Verification items for the finished model (mm, model axes). Give positions to 0.01 mm unless a question says otherwise; leave off trailing zeros. Loops run counter-clockwise (first coordinate to the right, second up) from the corner with the lowest first, then second, coordinate; pieces in that order, holes last. Notation, with made-up numbers: (43.5, 58) - (93.5, 58) arc R19 cw to (93.5, 95) - close; hole circle Ø6 at (-3, 67.5). An arc over 180 degrees is marked (long way). One line per question, with ' | ' between items. Start each with the question number.
1. Depth check by flat-ended pin: pin 1 Ø1.5 at (x, z) = (-42.5, -1) entering from +Y; pin 2 Ø9 at (x, y) = (-34, -12.5) entering from -Z; pin 3 Ø3 at (x, z) = (49.5, -3) entering from -Y. Enter the tip coordinate at first touch or a pass-through.
2. Section check D-D, the plane y = -13.5. Enter the section's corners in (x, z).
3. Section check B-B, the plane x = -34. Enter the section's corners in (y, z).
4. Section check A-A, the plane y = -22.5. Enter the section's corners in (x, z), then the cut area to 3 significant figures.
5. Section check C-C, the plane z = -2. Enter the section's corners in (x, y), then the cut area to 3 significant figures.
6. Thickness scan on line 1 along Y through (x, z) = (59.5, 0.85); line 2 along X through (y, z) = (-12.5, 1.55); line 3 along X through (y, z) = (-34.5, 1.4). Record the ranges inside material, lowest first. Write a range as from..to.
7. Mould release check, pull along Y, two halves, no side actions. Record for faces 1 (the face through (-60.933, 33.586, 0.986)), 2 (the face through (-1, -8, 0)), 3 (the face through (-36.77, -12.14, 0.99)), 4 (the face through (53.692, -7.663, -2.465)): +Y half, -Y half, draft (parallel to the pull), parting line (faces both ways), or undercut.
Autodesk Inventor part; units mm, degrees
ref_plane "YZ Plane" through (0, 0, 0) normal (1, 0, 0) x (0, 1, 0)
ref_plane "XZ Plane" through (0, 0, 0) normal (0, 1, 0) x (-1, 0, 0)
ref_plane "XY Plane" through (0, 0, 0) normal (0, 0, 1) x (1, 0, 0)
sketch "Sketch1" plane through (0, 0, 0) normal (0, 0, 1) x (1, 0, 0)
  line L0 (-62.5, 37.5) -> (62.5, 37.5)
  line L1 (62.5, 37.5) -> (62.5, -37.5)
  line L2 (62.5, -37.5) -> (-62.5, -37.5)
  line L3 (-62.5, -37.5) -> (-62.5, 37.5)
  point P0 (0, 0)
  point P1 (-62.5, 0)
  point P2 (0, 37.5)
  dimension "d0" = 125
  dimension "d1" = 75
extrude "Extrusion1" add sketch "Sketch1" along normal blind 2
sketch "Sketch2" plane through (0, 0, 2) normal (0, 0, 1) x (1, 0, 0)
  line L0 (-62.5, -37.5) -> (62.5, -37.5)
  line L1 (62.5, -37.5) -> (62.5, 37.5)
  line L2 (62.5, 37.5) -> (-62.5, 37.5)
  line L3 (-62.5, 37.5) -> (-62.5, -37.5)
  line L4 (-59.5, 34.5) -> (59.5, 34.5)
  line L5 (59.5, 34.5) -> (59.5, -34.5)
  line L6 (59.5, -34.5) -> (-59.5, -34.5)
  line L7 (-59.5, -34.5) -> (-59.5, 34.5)
  point P0 (0, 0)
  dimension "d4" = 3
hole "Hole1" at (-59.5, 34.5, 2) at (59.5, 34.5, 2) at (-59.5, -34.5, 2) at (59.5, -34.5, 2) direction (0, 0, -1) diameter 3.4 end through all
fillet "Fillet1" radius 2 4 edges at (-62.5, 37.5, 1) (-62.5, -37.5, 1) (62.5, -37.5, 1) (62.5, 37.5, 1)
sketch "Sketch3" plane through (0, 0, 2) normal (0, 0, 1) x (1, 0, 0)
  line L0 (18.5, 12.5) -> (45.5, 12.5)
  line L1 (45.5, 12.5) -> (45.5, -27.5)
  line L2 (45.5, -27.5) -> (18.5, -27.5)
  line L3 (18.5, -27.5) -> (18.5, 12.5)
  line L4 (62.5, -35.5) -> (62.5, 35.5)
  line L5 (60.5, 37.5) -> (-60.5, 37.5)
  point P0 (0, 0)
  dimension "d13" = 27
  dimension "d14" = 40
  dimension "d16" = 17
  dimension "d73" = 25
extrude "Extrusion2" cut sketch "Sketch3" against normal through all
fillet "Fillet2" radius 1.5 4 edges at (18.5, -27.5, 1) (18.5, 12.5, 1) (45.5, 12.5, 1) (45.5, -27.5, 1)
sketch "Sketch4" plane through (0, 0, 2) normal (0, 0, 1) x (1, 0, 0)
  line L0 (44, 12.5) -> (20, 12.5)
  line L1 (44, -27.5) -> (20, -27.5)
  line L2 (18.5, -26) -> (18.5, 11)
  line L3 (20, 12.5) -> (44, 12.5)
  line L4 (45.5, 11) -> (45.5, -26)
  line L5 (14.0041, -17.1435) -> (14.0041, 2.1435)
  line L6 (49.9959, 2.1435) -> (49.9959, -17.1435)
  line L7 (32, 12.5) -> (32, -27.5)
  point P0 (0, 0)
  point P1 (14.0041, -7.5)
  point P2 (49.9959, -7.5)
  point P3 (18.5, -7.5)
  point P4 (45.5, -7.5)
  dimension "d21" = 35.9918
hole "Hole2" at (14.0041, -7.5, 2) at (49.9959, -7.5, 2) direction (0, 0, -1) diameter 3.4 depth 6 tip angle 118
sketch "Sketch6" plane through (0, 0, 2) normal (0, 0, 1) x (1, 0, 0)
  circle A0 centre (-0.5, 10.5) radius 12.75
  line L0 (-11.4, 17.1146) -> (-11.4, 3.8854)
  line L1 (-62.5, 35.5) -> (-62.5, -35.5)
  line L2 (60.5, 37.5) -> (-60.5, 37.5)
  point P0 (0, 0)
  dimension "d35" = 25.5
  dimension "d36" = 10.9
  dimension "d74" = 62
  dimension "d75" = 27
extrude "Extrusion4" cut sketch "Sketch6" against normal blind 10 contours A0 L0 picked at (-2.2841, 10.5)
sketch "Sketch7" plane through (0, 0, 2) normal (0, 0, 1) x (1, 0, 0)
  line L0 (-47.5, -22.5) -> (6.5, -22.5)
  line L1 (-62.5, 35.5) -> (-62.5, -35.5)
  line L2 (-60.5, -37.5) -> (60.5, -37.5)
  line L3 (-34, -12.5) -> (-7, -12.5)
  point P0 (0, 0)
  point P1 (-20.5, -22.5)
  point P2 (-20.5, -12.5)
  dimension "d40" = 54
  dimension "d43" = 15
  dimension "d56" = 15
  dimension "d57" = 10
  dimension "d58" = 27
hole "Hole3" at (-47.5, -22.5, 2) at (6.5, -22.5, 2) at (-20.5, -22.5, 2) at (-34, -12.5, 2) at (-7, -12.5, 2) direction (0, 0, -1) diameter 5.588 end through all
sketch "Sketch8" plane through (0, 0, 0) normal (0, 0, -1) x (-1, 0, 0)
  circle A0 centre (-49.9959, -7.5) radius 1.7
  circle A1 centre (-14.0041, -7.5) radius 1.7
  circle A2 centre (-49.9959, -7.5) radius 3.7
  circle A3 centre (-14.0041, -7.5) radius 3.7
  point P0 (0, 0)
  dimension "d52" = 2
  dimension "d53" = 2
extrude "Extrusion5" add sketch "Sketch8" along normal blind 5
sketch "Sketch9" plane through (0, 0, 2) normal (0, 0, 1) x (1, 0, 0)
  circle A0 centre (-35.5, 10.5) radius 16.47
  line L0 (60.5, 37.5) -> (-60.5, 37.5)
  line L1 (-62.5, 35.5) -> (-62.5, -35.5)
  line L2 (-50.18, 25.18) -> (-20.82, 25.18)
  line L3 (-20.82, 25.18) -> (-20.82, -4.18)
  line L4 (-20.82, -4.18) -> (-50.18, -4.18)
  line L5 (-50.18, -4.18) -> (-50.18, 25.18)
  point P0 (0, 0)
  point P1 (-20.82, 10.5)
  point P2 (-35.5, 25.18)
  dimension "d59" = 32.94
  dimension "d60" = 27
  dimension "d61" = 27
  dimension "d62" = 29.36
  dimension "d63" = 29.36
extrude "Extrusion6" cut sketch "Sketch9" against normal blind 10 contours A0 L3 | L3 A0 L4 L5 L2 | L2 A0 | A0 L4 | L5 A0
hole "Hole4" at (-50.18, 25.18, 2) at (-20.82, 25.18, 2) at (-50.18, -4.18, 2) at (-20.82, -4.18, 2) direction (0, 0, -1) diameter 3.25 end through all
properties part number "LI0011-IO SHIELD"
Results list:
1) pin 1: through | pin 2: z = 0 | pin 3: y = -11.2
2) outline: (-62.5, 0) - (-36.61, 0) - (-36.61, 2) - (-62.5, 2) - close; (-31.39, 0) - (-9.61, 0) - (-9.61, 2) - (-31.39, 2) - close; (-4.39, 0) - (18.5, 0) - (18.5, 2) - (-4.39, 2) - close; (45.5, 0) - (62.5, 0) - (62.5, 2) - (45.5, 2) - close
3) outline: (-37.5, 0) - (-15.29, 0) - (-15.29, 2) - (-37.5, 2) - close; (-9.71, 0) - (-5.9, 0) - (-5.9, 2) - (-9.71, 2) - close; (26.9, 0) - (37.5, 0) - (37.5, 2) - (26.9, 2) - close
4) outline: (-62.5, 0) - (-50.29, 0) - (-50.29, 2) - (-62.5, 2) - close; (-44.71, 0) - (-23.29, 0) - (-23.29, 2) - (-44.71, 2) - close; (-17.71, 0) - (3.71, 0) - (3.71, 2) - (-17.71, 2) - close; (9.29, 0) - (18.5, 0) - (18.5, 2) - (9.29, 2) - close; (45.5, 0) - (62.5, 0) - (62.5, 2) - (45.5, 2) - close | area: 162 mm²
5) outline: circle Ø7.4 at (14, -7.5); circle Ø7.4 at (50, -7.5); hole circle Ø3.4 at (14, -7.5); hole circle Ø3.4 at (50, -7.5) | area: 67.9 mm²
6) line 1: -37.5..-36.2, -32.8..32.8, 36.2..37.5 | line 2: -62.5..-36.79, -31.21..-9.79, -4.21..18.5, 45.5..62.5 | line 3: -62.5..-61.2, -57.8..57.8, 61.2..62.5
7) face 1: undercut | face 2: draft | face 3: undercut | face 4: parting line
